The model under review builds one solid part; all positions refer to its coordinate system, in mm. A direction names the side the tool comes from. Give positions to 0.01 mm unless a question says otherwise; leave off trailing zeros. Loops run counter-clockwise (first coordinate to the right, second up) from the corner with the lowest first, then second, coordinate; pieces in that order, holes last. Notation, with made-up numbers: (82.25, 35.25) - (97.25, 35.25) arc R18 cw to (97.25, 53.25) - close; hole circle Ø5 at (33.5, 86). An arc over 180 degrees is marked (long way). Answer as a JSON object with one key per item and string values.
from build123d import *

# Parameters (mm, degrees)
F1_DEPTH = 15
F3_D     = 3.3


with BuildPart() as f1:
    # F0 (on Front) → F1 (new body, symmetric)
    with BuildSketch(Plane.XZ):
        with BuildLine():
            Line((-5.4519269615, 0), (0, 0))
            Line((0, 0), (0, 3))
            ThreePointArc((0, 3), (-7.5, 10.5), (0, 18))
            Line((0, 18), (0, 21.5))
            Line((0, 21.5), (-3.4802674782, 21.5))
            Line((-3.4802674782, 21.5), (-9.6111802198, 17.5))
            Line((-9.6111802198, 17.5), (-16.5, 17.5))
            Line((-16.5, 17.5), (-16.5, 6.8754809164))
            Line((-16.5, 6.8754809164), (-17, 5.5))
            Line((-17, 5.5), (-17, -0.5))
            Line((-17, -0.5), (-9.6111802198, -0.5))
            Line((-9.6111802198, -0.5), (-5.4519269615, 0))
        make_face()
        with BuildLine():
            Line((0, 3), (0, 0))
            Line((0, 0), (5.4519269615, 0))
            Line((5.4519269615, 0), (9.6111802198, -0.5))
            Line((9.6111802198, -0.5), (17, -0.5))
            Line((17, -0.5), (17, 5.5))
            Line((17, 5.5), (16.5, 6.8754809164))
            Line((16.5, 6.8754809164), (16.5, 17.5))
            Line((16.5, 17.5), (9.6111802198, 17.5))
            Line((9.6111802198, 17.5), (3.4802674782, 21.5))
            Line((3.4802674782, 21.5), (0, 21.5))
            Line((0, 21.5), (0, 18))
            ThreePointArc((0, 18), (7.5, 10.5), (0, 3))
        make_face()
    extrude(amount=F1_DEPTH, both=True)

    # F3 (through all)
    with Locations(Plane(origin=(0, 0, -0.5), x_dir=(1, 0, 0), z_dir=(0, 0, -1))):
        with Locations((-13.4, 10.7), (-13.4, -10.7), (13.4, -10.7), (13.4, 10.7)):
            Hole(F3_D / 2)


solid = f1.part
Q1. The part is to be moulded in two halves that separate along Z. For faces 4 (the face through (0, 0, 3)), 5 (the face through (-4, -15, 3)), 6 (the face through (-7.561, -0.21, -0.253)), say which applies: +Z half, -Z half, draft (parallel to the pull), parting line (faces both ways), or undercut.
Results:
{"face 4": "undercut", "face 5": "draft", "face 6": "-Z half"}
Q2. Consider section D-D, the plane y = -4.75. State the section outline as (x, z) points.
Results:
{"outline": "(-17, -0.5) - (-9.61, -0.5) - (-5.45, 0) - (5.45, 0) - (9.61, -0.5) - (17, -0.5) - (17, 5.5) - (16.5, 6.88) - (16.5, 17.5) - (9.61, 17.5) - (3.48, 21.5) - (-3.48, 21.5) - (-9.61, 17.5) - (-16.5, 17.5) - (-16.5, 6.88) - (-17, 5.5) - close; hole circle Ø15 at (0, 10.5)"}
Q3. Consider section C-C, the plane z = 13.5. State the section outline as (x, y) points, plus the area to 3 significant figures.
Results:
{"outline": "(-16.5, -15) - (-6.87, -15) - (-6.87, 15) - (-16.5, 15) - close; (6.87, -15) - (16.5, -15) - (16.5, 15) - (6.87, 15) - close; hole circle Ø3.3 at (-13.4, -10.7); hole circle Ø3.3 at (-13.4, 10.7); hole circle Ø3.3 at (13.4, -10.7); hole circle Ø3.3 at (13.4, 10.7)", "area": "543 mm^2"}
Q4. To check wall thickness, follow probe 1 along Y at (x, z) = (-13.4, 7.25); probe 2 along X at (y, z) = (-10.7, 10.5); probe 3 along Y at (x, z) = (-14, 11.5). State the ranges of each line that lie inside material, in increasing order. Write a range as [from, to].
Results:
{"probe 1": "y = [-15, -12.35], [-9.05, 9.05], [12.35, 15]", "probe 2": "x = [-16.5, -15.05], [-11.75, -7.5], [7.5, 11.75], [15.05, 16.5]", "probe 3": "y = [-15, -12.24], [-9.16, 9.16], [12.24, 15]"}
Q5. Consider section B-B, the plane x = 0. State the section outline as (y, z) points.
Results:
{"outline": "(-15, 0) - (15, 0) - (15, 3) - (-15, 3) - close; (-15, 18) - (15, 18) - (15, 21.5) - (-15, 21.5) - close"}
Q6. For faces 1 (the face through (0, 0, 0)), 2 (the face through (-13, 0, 17.5)), 3 (the face through (16.5, 0, 12)), list the 3-axis set-ups (+Z, -Z, +X, -X, +Y, -Y) from which the entire face can be reached by the end or side of a thin tool; tool diameter is ignored.
Results:
{"face 1": "-Z, +Y, -Y", "face 2": "+Z, -X, +Y, -Y", "face 3": "+Z, +X, +Y, -Y"}
Q7. Consider section A-A, the plane y = 10.7. State the section outline as (x, z) points.
Results:
{"outline": "(-17, -0.5) - (-15.05, -0.5) - (-15.05, 17.5) - (-16.5, 17.5) - (-16.5, 6.88) - (-17, 5.5) - close; (-11.75, -0.5) - (-9.61, -0.5) - (-5.45, 0) - (5.45, 0) - (9.61, -0.5) - (11.75, -0.5) - (11.75, 17.5) - (9.61, 17.5) - (3.48, 21.5) - (-3.48, 21.5) - (-9.61, 17.5) - (-11.75, 17.5) - close; (15.05, -0.5) - (17, -0.5) - (17, 5.5) - (16.5, 6.88) - (16.5, 17.5) - (15.05, 17.5) - close; hole circle Ø15 at (0, 10.5)"}
Q8. Clearance check with flat-ended pins moving along their axes: pin 1 Ø3.5 at (x, y) = (-12.5, 6.5) entering from +Z; pin 2 Ø10 at (y, z) = (1.5, 9.5) entering from +X; pin 3 Ø4 at (y, z) = (10, 16.5) entering from -X; pin 4 Ø1.5 at (x, y) = (-9, -5) entering from +Z. State where each tip first meets the part, or that it passes through.
Results:
{"pin 1": "stops at z = 17.5", "pin 2": "stops at x = 17", "pin 3": "stops at x = -16.5", "pin 4": "stops at z = 18.39"}
